Answer from the drawing. Dimensions are ordinates in mm from the lowest x, y and z of the part. A direction names the side the tool comes from. Give positions to 0.01 mm unless a question says otherwise; leave off trailing zeros. Order: outer loops, then holes, each group sorted by start corner. A loop starts at its lowest first (then second) coordinate and runs counter-clockwise, first axis right, second up. Notation, with made-up numbers: (10, 87) -> (45, 87) arc R20 ccw to (45, 116) -> close; hole circle Ø6 at (78.25, 10.25). An arc over 180 degrees is marked (long way). One line per question, with ' | ' between items. Start each with the question number.
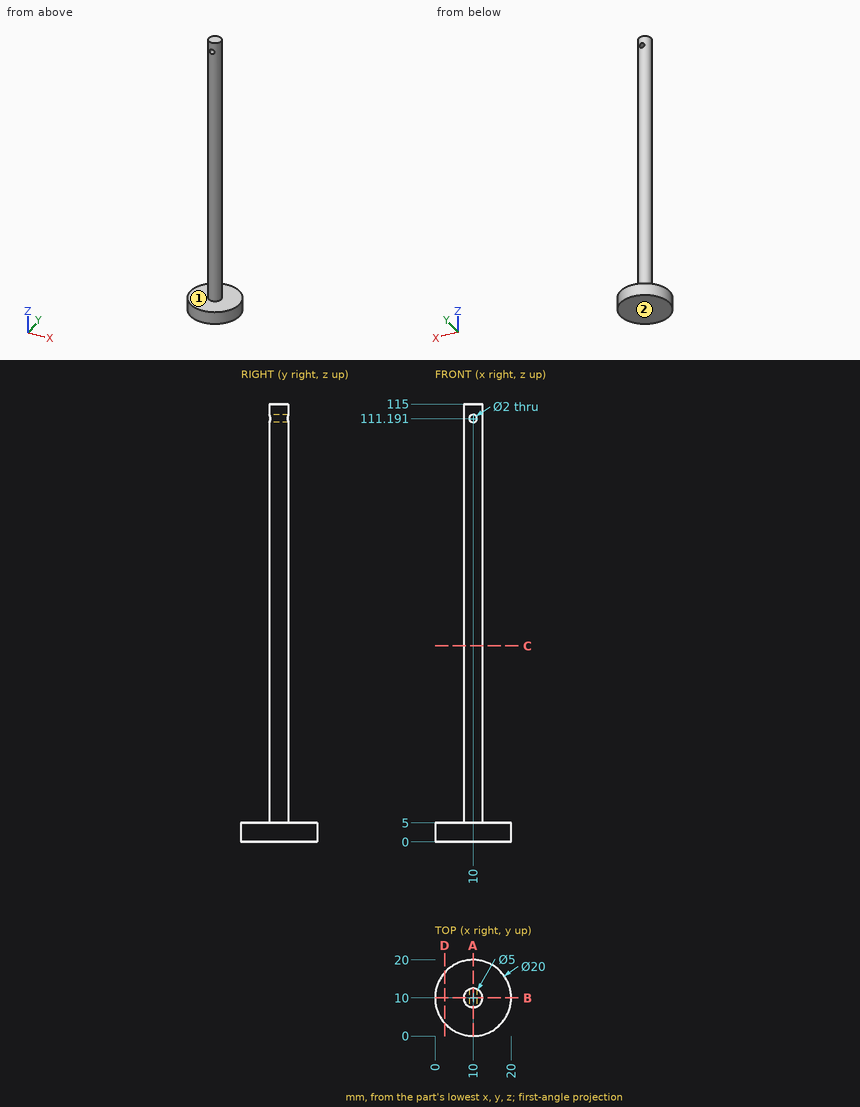
(1) Consider line 1 (Z direction, x = 10, y = 8.6); line 2 (Z direction, x = 6.75, y = 16.25); line 3 (X direction, y = 10.25, z = 53). Determine where each line is inside the solid, lowest interval first.
(2) The part is cut by section D-D on x = 2.5. Determine the outline of the cut face in (y, z) (1 decimal).
(3) The part is cut by section A-A on x = 10. Determine the outline of the cut face in (y, z).
(4) The part is cut by section C-C on z = 51.5. Determine the outline of the cut face in (x, y).
(5) For the marked faces 1 and 2, determine the directions among +Z, -Z, +X, -X, +Y, -Y from which every point of the face is accessible in a straight line to the end or side of a thin tool.
(6) The part is cut by section B-B on y = 10. Determine the outline of the cut face in (x, z), plus the area to 3 significant figures.
(7) Given P1, Ø10, axis at x = 16.5, y = 17.5, coming from the -Z side; P2, Ø8, axis at x = 14.5, y = 3.5, coming from the +Z side; P3, Ø5, axis at y = 13, z = 102, coming from the -X side; P4, Ø2.5, axis at x = 10, z = 111.19, coming from the -Y side, each flat-ended and moving along its own axis, determine where each tip first touches the part or whether it passes through.
Result sheet:
1) line 1: z = 0 to 110.19, 112.19 to 115 | line 2: z = 0 to 5 | line 3: x = 7.51 to 12.49
2) outline: (3.4, 0) -> (16.6, 0) -> (16.6, 5) -> (3.4, 5) -> close
3) outline: (0, 0) -> (20, 0) -> (20, 5) -> (12.5, 5) -> (12.5, 110.19) -> (7.5, 110.19) -> (7.5, 5) -> (0, 5) -> close; (7.5, 112.19) -> (12.5, 112.19) -> (12.5, 115) -> (7.5, 115) -> close
4) outline: circle Ø5 at (10, 10)
5) face 1: +Z | face 2: -Z, +X, -X, +Y, -Y
6) outline: (0, 0) -> (20, 0) -> (20, 5) -> (12.5, 5) -> (12.5, 115) -> (7.5, 115) -> (7.5, 5) -> (0, 5) -> close; hole circle Ø2 at (10, 111.19) | area: 647 mm^2
7) P1: stops at z = 0 | P2: stops at z = 5 | P3: stops at x = 7.55 | P4: stops at y = 7.5
